from build123d import *

# Parameters (mm, degrees)
F0_W     = 58.757578
F0_H     = 12
F0_W_2   = 50
F0_H_2   = 5.2
F1_DEPTH = 6
F0_W_3   = 6.612889
F2_DEPTH = 20
F3_R     = 2
F4_R     = 2
F5_R     = 2
F6_R     = 2
F7_R     = 5


with BuildPart() as f1:
    # F0 (on Top) → F1 (new body)
    with BuildSketch(Plane.XY):
        with Locations((13.568355, 32.723509)):
            Rectangle(F0_W, F0_H)
        with Locations((12.947144, 32.723509)):
            Rectangle(F0_W_2, F0_H_2, mode=Mode.SUBTRACT)
    extrude(amount=F1_DEPTH)

    # F0 (on Top) → F2 (join)
    with BuildSketch(Plane.XY):
        with Locations((-19.116878, 32.723509)):
            Rectangle(F0_W_3, F0_H)
    extrude(amount=F2_DEPTH)

    # F3
    f3_edges = [f1.edges().sort_by_distance(p)[0] for p in [
        (42.947144, 26.723509, 3),
    ]]
    fillet(f3_edges, radius=F3_R)

    # F4
    f4_edges = [f1.edges().sort_by_distance(p)[0] for p in [
        (42.947144, 38.723509, 3),
    ]]
    fillet(f4_edges, radius=F4_R)

    # F5
    f5_edges = [f1.edges().sort_by_distance(p)[0] for p in [
        (-12.052856, 35.323509, 3),
        (37.947144, 35.323509, 3),
        (37.947144, 30.123509, 3),
        (-12.052856, 30.123509, 3),
    ]]
    fillet(f5_edges, radius=F5_R)

    # F6
    f6_edges = [f1.edges().sort_by_distance(p)[0] for p in [
        (-22.423323, 38.723509, 10),
        (-22.423323, 26.723509, 10),
    ]]
    fillet(f6_edges, radius=F6_R)

    # F7
    f7_edges = [f1.edges().sort_by_distance(p)[0] for p in [
        (-15.810434, 32.723509, 20),
    ]]
    fillet(f7_edges, radius=F7_R)


solid = f1.part
The model under review builds one solid part; all positions refer to its coordinate system, in mm. A direction names the side the tool comes from. Round coordinates to 2 decimals unless told otherwise and drop trailing zeros. Loops run counter-clockwise (first coordinate to the right, second up) from the corner with the lowest first, then second, coordinate; pieces in that order, holes last. Notation, with made-up numbers: (13.5, -36) -> (68.5, -36) arc R22 ccw to (68.5, -28) -> close; hole circle Ø5 at (-7.5, 41.5). An arc over 180 degrees is marked (long way). Answer as CSV lines item,"result".
1) Tool access review of faces 1 (the face through (37.4, 34.7, 3)), 2 (the face through (13.2, 35.5, 6)), 3 (the face through (-22.423, 33, 10)): name each direction out of +Z, -Z, +X, -X, +Y, -Y from which nothing blocks a thin tool from reaching the whole face with its end or side.
Geometry results:
face 1,"+Z, -Z"
face 2,"+Z, +X, +Y, -Y"
face 3,"+Z, -Z, -X, +Y, -Y"
2) Add section C-C on y = 31. Write out the cut boundary in (x, z), plus the area to 3 significant figures.
Geometry results:
outline,"(-22.42, 0) -> (-11.71, 0) -> (-11.71, 6) -> (-15.81, 6) -> (-15.81, 15) arc R5 ccw to (-20.81, 20) -> (-22.42, 20) -> close; (37.6, 0) -> (42.95, 0) -> (42.95, 6) -> (37.6, 6) -> close"
area,"184 mm²"
3) Add section A-A on z = 2.5. Write out the cut boundary in (x, y).
Geometry results:
outline,"(-22.42, 28.72) arc R2 ccw to (-20.42, 26.72) -> (40.95, 26.72) arc R2 ccw to (42.95, 28.72) -> (42.95, 36.72) arc R2 ccw to (40.95, 38.72) -> (-20.42, 38.72) arc R2 ccw to (-22.42, 36.72) -> close; hole (-12.05, 32.12) arc R2 ccw to (-10.05, 30.12) -> (35.95, 30.12) arc R2 ccw to (37.95, 32.12) -> (37.95, 33.32) arc R2 ccw to (35.95, 35.32) -> (-10.05, 35.32) arc R2 ccw to (-12.05, 33.32) -> close"
4) Add section D-D on y = 37.75. Write out the cut boundary in (x, z).
Geometry results:
outline,"(-22.14, 0) -> (42.66, 0) -> (42.66, 6) -> (-15.81, 6) -> (-15.81, 15) arc R5 ccw to (-20.81, 20) -> (-22.14, 20) -> close"
5) For P1, Ø1, axis at x = -8, y = 28.5, coming from the -Z side; P2, Ø3.5, axis at x = 25, y = 34, coming from the +Z side; P3, Ø2.5, axis at y = 34.5, z = 9, coming from the +X side, all flat-tipped, find the tip position at first contact; note any pin that passes through.
Geometry results:
P1,"stops at z = 0"
P2,"stops at z = 6"
P3,"stops at x = -15.81"
6) Add section B-B on x = 12. Write out the cut boundary in (y, z), plus the area to 3 significant figures.
Geometry results:
outline,"(26.72, 0) -> (30.12, 0) -> (30.12, 6) -> (26.72, 6) -> close; (35.32, 0) -> (38.72, 0) -> (38.72, 6) -> (35.32, 6) -> close"
area,"40.8 mm²"
7) To check wall thickness, follow line 1 along X through (y, z) = (36.5, 7.75); line 2 along Y through (x, z) = (35.5, 1.25); line 3 along Z through (x, y) = (0, 28). State the ranges of each line that lie inside material, in increasing order. Write a range as from..to.
Geometry results:
line 1,"x = -22.42..-15.81"
line 2,"y = 26.72..30.12, 35.32..38.72"
line 3,"z = 0..6"
8) Draft analysis for pull direction X (two halves, no side actions). For faces 4 (the face through (-21.82, 27.29, 10.14)), 5 (the face through (37.346, 30.694, 3.042)), 6 (the face through (-15.81, 33, 10)), 7 (the face through (37.947, 33, 3)), state which applies: pulls with the +X half, pulls with the -X half, needs draft (parallel to the pull), parting line crosses it, or undercut.
Geometry results:
face 4,"pulls with the -X half"
face 5,"undercut"
face 6,"pulls with the +X half"
face 7,"undercut"
